For this review, use the dimensioned drawing (mm, ordinates from the lowest corner) and the shaded views. A direction names the side the tool comes from. Coordinates: 2 decimals unless noted, no trailing zeros. Write each loop counter-clockwise with the first axis right and the second up, starting at its lowest first coordinate (ties: lowest second). Pieces come first, ordered by that corner, then holes. Notation, with made-up numbers: (14, 87) - (46, 87) arc R28 cw to (46, 112) - close; hole circle Ø4 at (-5, 52.5). An arc over 180 degrees is marked (long way). Answer as a JSON object with one key per item and string values.
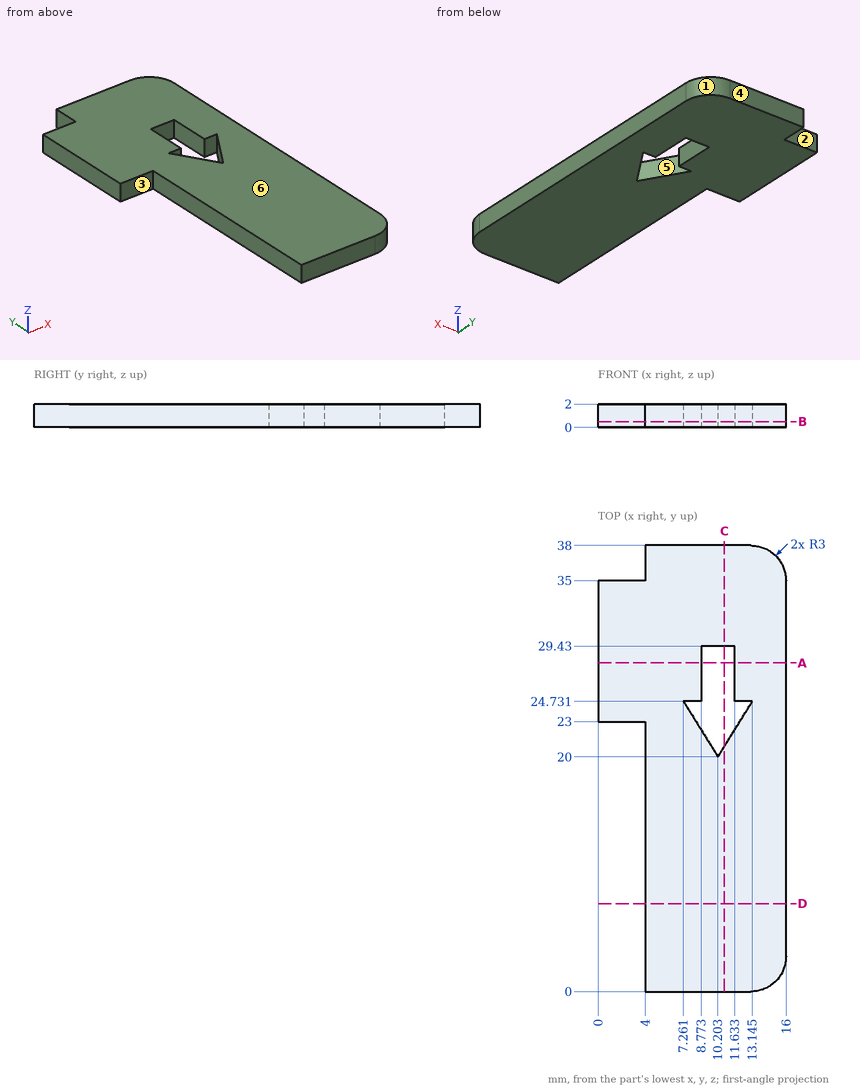
(1) Tool access review of the marked faces 1 and 2: name each direction out of +Z, -Z, +X, -X, +Y, -Y from which nothing blocks a thin tool from reaching the whole face with its end or side.
Solved:
{"face 1": "+Z, -Z, +X, +Y", "face 2": "+Z, -Z, -X, +Y"}
(2) Take a section at D-D, the plane y = 7.5. Write out the cut boundary in (x, z).
Solved:
{"outline": "(4, 0) - (16, 0) - (16, 2) - (4, 2) - close"}
(3) Take a section at A-A, the plane y = 28. Write out the cut boundary in (x, z).
Solved:
{"outline": "(0, 0) - (8.77, 0) - (8.77, 2) - (0, 2) - close; (11.63, 0) - (16, 0) - (16, 2) - (11.63, 2) - close"}
(4) To check wall thickness, follow line 1 (X direction, y = 26, z = 0.1); line 2 (Y direction, x = 2, z = 1.15); line 3 (Y direction, x = 9.75, z = 0.9). State the ranges of each line that lie inside material, in increasing order. Write a range as from..to.
Solved:
{"line 1": "x = 0..8.77, 11.63..16", "line 2": "y = 23..35", "line 3": "y = 0..20.73, 29.43..38"}
(5) Take a section at C-C, the plane x = 10.75. Write out the cut boundary in (y, z).
Solved:
{"outline": "(0, 0) - (20.88, 0) - (20.88, 2) - (0, 2) - close; (29.43, 0) - (38, 0) - (38, 2) - (29.43, 2) - close"}
(6) For pin 1 (0.6 mm diameter, centred on y = 7.5, z = 1, fed in from -X); pin 2 (0.6 mm diameter, centred on y = 27, z = 0.5, fed in from -X); pin 3 (0.6 mm diameter, centred on x = 2, z = 1, fed in from -Y), all flat-tipped, find the tip position at first contact; note any pin that passes through.
Solved:
{"pin 1": "stops at x = 4", "pin 2": "stops at x = 0", "pin 3": "stops at y = 23"}
(7) Take a section at B-B, the plane z = 0.5. Write out the cut boundary in (x, y) (1 decimal), and give its area (3 significant figures).
Solved:
{"outline": "(0, 23) - (4, 23) - (4, 0) - (13, 0) arc R3 ccw to (16, 3) - (16, 35) arc R3 ccw to (13, 38) - (4, 38) - (4, 35) - (0, 35) - close; hole (7.3, 24.7) - (10.2, 20) - (13.1, 24.7) - (11.6, 24.7) - (11.6, 29.4) - (8.8, 29.4) - (8.8, 24.7) - close", "area": "473 mm^2"}
(8) The part is to be moulded in two halves that separate along Y. For the marked faces 3, 4, 5 and 6, say which applies: pulls with the +Y half, pulls with the -Y half, needs draft (parallel to the pull), parting line crosses it, or undercut.
Solved:
{"face 3": "pulls with the -Y half", "face 4": "pulls with the +Y half", "face 5": "undercut", "face 6": "needs draft"}
